For this review, take the finished solid that the model builds, in its own axes (mm). A direction names the side the tool comes from. Give positions to 0.01 mm unless a question says otherwise; leave off trailing zeros. Order: outer loops, then holes, each group sorted by start corner. A loop starts at its lowest first (then second) coordinate and runs counter-clockwise, first axis right, second up. Notation, with made-up numbers: (-26, 47) - (18, 47) arc R24 ccw to (18, 74) - close; hole circle Ø7 at (59.25, 78.25). An arc over 180 degrees is marked (long way). Answer as a JSON object with one key per item and string values. Group by question number.
from build123d import *

# Parameters (mm, degrees)
SKETCH1_R            = 0.5
FRONT_FACE_EXT_DEPTH = 1
SKETCH2_W            = 1
SKETCH2_H            = 6.5
BOSS_EXTRUDE1_DEPTH  = 1.7874
SKETCH3_W            = 1
SKETCH3_H            = 1
BOSS_EXTRUDE2_DEPTH  = 1
SKETCH4_W            = 10.7874
SKETCH4_H            = 1
BOSS_EXTRUDE3_DEPTH  = 0.8


with BuildPart() as part:
    # Sketch1 → Front Face Ext (new body)
    with BuildSketch(Plane.XY):
        with BuildLine():
            Line((-3.75, -3.25), (-4.5, -3.25))
            Line((-4.5, -3.25), (-4.5, 3.25))
            Line((-4.5, 3.25), (4.5, 3.25))
            Line((4.5, 3.25), (4.5, -3.25))
            Line((4.5, -3.25), (-2.75, -3.25))
            ThreePointArc((-2.75, -3.25), (-3.25, -2.75), (-3.75, -3.25))
        make_face()
        with Locations((-2.5, 2.25)):
            Circle(SKETCH1_R, mode=Mode.SUBTRACT)
        with Locations((3.5, -0.25)):
            Circle(SKETCH1_R, mode=Mode.SUBTRACT)
    extrude(amount=FRONT_FACE_EXT_DEPTH)

    # Sketch2 → Boss-Extrude1 (add)
    with BuildSketch(Plane.ZY.offset(4.5)):
        with Locations((0.5, 0)):
            Rectangle(SKETCH2_W, SKETCH2_H)
    extrude(amount=BOSS_EXTRUDE1_DEPTH)

    # Sketch3 → Boss-Extrude2 (add)
    with BuildSketch(Plane.XY.offset(1)):
        with Locations((-5.7874, 2.75)):
            Rectangle(SKETCH3_W, SKETCH3_H)
        with Locations((-5.7874, -2.75)):
            Rectangle(SKETCH3_W, SKETCH3_H)
    extrude(amount=BOSS_EXTRUDE2_DEPTH)

    # Sketch4 → Boss-Extrude3 (add)
    with BuildSketch(Plane(origin=(0, 3.25, 0), x_dir=(1, 0, 0), z_dir=(0, 1, 0))):
        with Locations((-0.8937, -0.5)):
            Rectangle(SKETCH4_W, SKETCH4_H)
    extrude(amount=BOSS_EXTRUDE3_DEPTH)


solid = part.part
1) Mouldability with a two-part tool opening along Y and no side actions: class faces 1 (the face through (-5.287, -2.8, 1.5)), 2 (the face through (-2.565, 2.746, 0.493)), 3 (the face through (-1, 4.05, 0.5)) as released by +Y, released by -Y, zero draft, split by the parting line, or undercut.
2) For faces 4 (the face through (-5.8, 3.25, 1.5)), 5 (the face through (-5.8, 2.25, 1.5)), 6 (the face through (-6, -3, 2)), 7 (the face through (3, -0.23, 0.49)), 8 (the face through (-5.287, 2.7, 1.5)), list the 3-axis set-ups (+Z, -Z, +X, -X, +Y, -Y) from which the entire face can be reached by the end or side of a thin tool; tool diameter is ignored.
3) For pin 1 (1.1 mm diameter, centred on x = -6, z = 1.5, fed in from +Y); pin 2 (0.5 mm diameter, centred on y = -3, z = 1.5, fed in from +X), all flat-tipped, find the tip position at first contact; note any pin that passes through.
4) Consider section A-A (x = 3.5). Give the boundary of the cut face in (y, z).
5) For line 1 (Y direction, x = -2.5, z = 0.45); line 2 (X direction, y = 2.5, z = 1.7); line 3 (Z direction, x = -3.5, y = -2), list the stretches that pass through material, from the lowest coordinate up.
6) Consider section D-D (z = 0.6). Give the boundary of the cut face in (x, y).
7) Consider section B-B (z = 1.2). Give the boundary of the cut face in (x, y).
8) Consider section C-C (y = 2.5). Give the boundary of the cut face in (x, z).
Result set:
{
 "1": {"face 1": "zero draft", "face 2": "undercut", "face 3": "released by +Y"},
 "2": {"face 4": "+Z, +X, -X, +Y", "face 5": "+Z, +X, -X", "face 6": "+Z, +X, -X, +Y, -Y", "face 7": "+Z, -Z", "face 8": "+Z, +X, +Y, -Y"},
 "3": {"pin 1": "stops at y = 4.05", "pin 2": "stops at x = -5.29"},
 "4": {"outline": "(-3.25, 0) - (-0.75, 0) - (-0.75, 1) - (-3.25, 1) - close; (0.25, 0) - (4.05, 0) - (4.05, 1) - (0.25, 1) - close"},
 "5": {"line 1": "y = -3.25 to 1.75, 2.75 to 4.05", "line 2": "x = -6.29 to -5.29", "line 3": "z = 0 to 1"},
 "6": {"outline": "(-6.29, -3.25) - (-3.75, -3.25) arc R0.5 cw to (-2.75, -3.25) - (4.5, -3.25) - (4.5, 4.05) - (-6.29, 4.05) - close; hole circle Ø1 at (-2.5, 2.25); hole circle Ø1 at (3.5, -0.25)"},
 "7": {"outline": "(-6.29, -3.25) - (-5.29, -3.25) - (-5.29, -2.25) - (-6.29, -2.25) - close; (-6.29, 2.25) - (-5.29, 2.25) - (-5.29, 3.25) - (-6.29, 3.25) - close"},
 "8": {"outline": "(-6.29, 0) - (-2.93, 0) - (-2.93, 1) - (-5.29, 1) - (-5.29, 2) - (-6.29, 2) - close; (-2.07, 0) - (4.5, 0) - (4.5, 1) - (-2.07, 1) - close"}
}
